Source: CAD feature listing. Evaluate the final solid. Frame: model axes, mm. Face numbers are marked on the shaded views. A direction names the side the tool comes from. Round coordinates to 2 decimals unless told otherwise and drop trailing zeros. Loops run counter-clockwise (first coordinate to the right, second up) from the corner with the lowest first, then second, coordinate; pieces in that order, holes last. Notation, with made-up numbers: M -28,46 L -7,46 A25 cw -7,81 Z; hole C 15.25,71.5 d5. An arc over 180 degrees is marked long. Answer as a JSON object with one key per item and string values.
from build123d import *

# Parameters (mm, degrees)
BOSS_EXTRUDE1_DEPTH  = 14
SKETCH20_W           = 45
SKETCH20_H           = 14
BOSS_EXTRUDE10_DEPTH = 5
SKETCH21_R           = 2.65
CUT_EXTRUDE13_DEPTH  = 5
SKETCH22_W           = 5
SKETCH22_H           = 4
CUT_EXTRUDE14_DEPTH  = 62.814237842
SKETCH23_R           = 2.65
BOSS_EXTRUDE11_DEPTH = 5
SKETCH24_W           = 25
SKETCH24_H           = 7
CUT_EXTRUDE15_DEPTH  = 3
CUT_EXTRUDE16_REACH  = 68.31
SKETCH25_W           = 12
SKETCH25_H           = 7
CUT_EXTRUDE17_REACH  = 70.644
SKETCH26_W           = 5
SKETCH26_H           = 14


with BuildPart() as part:
    # Sketch1 → Boss-Extrude1 (new body)
    with BuildSketch(Plane(origin=(0, 0, 0), x_dir=(1, 0, 0), z_dir=(0, 1, 0))):
        Polygon((6.589095597, 0), (10, 0), (10, 4), (40, 4), (40, 9), (11.589095597, 9), (0, 9), (0, 0), align=None)
    extrude(amount=BOSS_EXTRUDE1_DEPTH)

    # Sketch20 → Boss-Extrude10 (add)
    with BuildSketch(Plane.ZY):
        with Locations((22.5, 7)):
            Rectangle(SKETCH20_W, SKETCH20_H)
    extrude(amount=-BOSS_EXTRUDE10_DEPTH)

    # Sketch21 → Cut-Extrude13 (cut)
    with BuildSketch(Plane.ZY):
        with Locations((0, 7)):
            Circle(SKETCH21_R)
        with Locations((8, 7)):
            Circle(SKETCH21_R)
        with Locations((16, 7)):
            Circle(SKETCH21_R)
        with Locations((24, 7)):
            Circle(SKETCH21_R)
        with Locations((32, 7)):
            Circle(SKETCH21_R)
        with Locations((40, 7)):
            Circle(SKETCH21_R)
    extrude(amount=-CUT_EXTRUDE13_DEPTH, mode=Mode.SUBTRACT)

    # Sketch22 → Cut-Extrude14 (cut, through all)
    with BuildSketch(Plane(origin=(0, 14, 0), x_dir=(1, 0, 0), z_dir=(0, 1, 0))):
        with Locations((7.5, 2)):
            Rectangle(SKETCH22_W, SKETCH22_H)
    extrude(amount=-CUT_EXTRUDE14_DEPTH, mode=Mode.SUBTRACT)

    # Sketch23 → Boss-Extrude11 (add)
    with BuildSketch(Plane.ZY):
        with Locations((0, 7)):
            Circle(SKETCH23_R)
    extrude(amount=-BOSS_EXTRUDE11_DEPTH)

    # Sketch24 → Cut-Extrude15 (cut)
    with BuildSketch(Plane(origin=(0, 0, -9), x_dir=(-1, 0, 0), z_dir=(0, 0, -1))):
        with Locations((-20.5, 7)):
            Rectangle(SKETCH24_W, SKETCH24_H)
    extrude(amount=-CUT_EXTRUDE15_DEPTH, mode=Mode.SUBTRACT)

    # Sketch25 → Cut-Extrude16 (cut, up to next)
    with BuildSketch(Plane(origin=(0, 0, -6), x_dir=(-1, 0, 0), z_dir=(0, 0, -1)), mode=Mode.PRIVATE) as cut_extrude16_sk1:
        with Locations((-20.5, 7)):
            Rectangle(SKETCH25_W, SKETCH25_H)
    cut_extrude16_tool1 = extrude(cut_extrude16_sk1.sketch, amount=-CUT_EXTRUDE16_REACH, mode=Mode.PRIVATE) & part.part
    add(cut_extrude16_tool1.solids().sort_by_distance((20.5, 7, -6))[0], mode=Mode.SUBTRACT)

    # Sketch26 → Cut-Extrude17 (cut, up to next)
    with BuildSketch(Plane(origin=(0, 0, -9), x_dir=(-1, 0, 0), z_dir=(0, 0, -1)), mode=Mode.PRIVATE) as cut_extrude17_sk1:
        with Locations((-37.5, 7)):
            Rectangle(SKETCH26_W, SKETCH26_H)
    cut_extrude17_tool1 = extrude(cut_extrude17_sk1.sketch, amount=-CUT_EXTRUDE17_REACH, mode=Mode.PRIVATE) & part.part
    add(cut_extrude17_tool1.solids().sort_by_distance((37.5, 7, -9))[0], mode=Mode.SUBTRACT)


solid = part.part
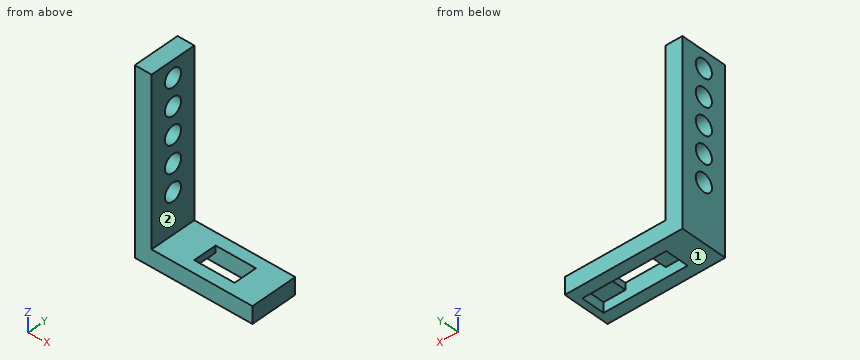
Item 1: Access query for the marked faces 1 and 2. Directions: +Z, -Z, +X, -X, +Y, -Y. A direction counts if a zero-diameter tool reaches every point of the face in a straight line with its end or side. Return the directions, or none.
Answer sheet:
{"face 1": "-Z, +X, -X, +Y, -Y", "face 2": "+Z, +X, +Y, -Y"}
Item 2: Contact query for flat-ended pins moving along their axis: pin 1 Ø4 at (y, z) = (6, 11.5) entering from +X; pin 2 Ø2 at (x, y) = (12, 8.5) entering from -Z. Output: stop coordinate, or through.
Answer sheet:
{"pin 1": "stops at x = 5", "pin 2": "stops at z = -6"}
Item 3: Section C-C on z = 32. Return the cut outline in (x, y), then the cut area to 3 significant figures.
Answer sheet:
{"outline": "M 0,0 L 5,0 L 5,4.35 L 0,4.35 Z; M 0,9.65 L 5,9.65 L 5,14 L 0,14 Z", "area": "43.5 mm²"}
Item 4: Section B-B on y = 7. Give the number of separate pieces and of enclosed holes in the cut face, then the cut area to 4 significant figures.
Answer sheet:
{"separate pieces": "7", "enclosed holes": "0", "area": "188.5 mm²"}
Item 5: Section A-A on x = 23. Return the cut outline in (y, z), then the cut area to 3 significant figures.
Answer sheet:
{"outline": "M 0,-9 L 3.5,-9 L 3.5,-4 L 0,-4 Z; M 10.5,-9 L 14,-9 L 14,-4 L 10.5,-4 Z", "area": "35.0 mm²"}
Item 6: Line query: probe 1 along Y at (x, z) = (3.95, 16); probe 2 along Z at (x, y) = (22.5, 12.5); probe 3 along X at (y, z) = (10, 8.5). Output: solid intervals per line, ascending. Write a range as from..to.
Answer sheet:
{"probe 1": "y = 0..4.35, 9.65..14", "probe 2": "z = -9..-4", "probe 3": "x = 0..5"}
Item 7: Section D-D on x = 9. Return the cut outline in (y, z), then the cut area to 3 significant figures.
Answer sheet:
{"outline": "M 0,-9 L 3.5,-9 L 3.5,-6 L 10.5,-6 L 10.5,-9 L 14,-9 L 14,-4 L 0,-4 Z", "area": "49.0 mm²"}
